Design review of the part built by this model. Coordinates are the model's own, in mm. A direction names the side the tool comes from. Give positions to 0.01 mm unless a question says otherwise; leave off trailing zeros. Loops run counter-clockwise (first coordinate to the right, second up) from the corner with the lowest first, then second, coordinate; pieces in that order, holes last. Notation, with made-up numbers: (-17.5, 32.25) -> (34.5, 32.25) arc R19 cw to (34.5, 62.25) -> close; hole circle Ø7 at (77.25, 4.25). An arc over 180 degrees is marked (long way). Answer in a Markdown table with one row per item. Add a question column.
(1) Draft analysis for pull direction X (two halves, no side actions). For faces 1 (the flat face through (9.15, 0, 1)), 2 (the flat face through (-0.394, -5.406, 0.74)), 3 (the flat face through (0, -12.3, 1)), state which applies: +X half, -X half, draft (parallel to the pull), parting line (faces both ways), or undercut.
(2) Consider section B-B on z = 0.4. Write out the cut boundary in (x, y).
(3) For line 1 (Y direction, x = 0.75, z = 1.35); line 2 (X direction, y = -6.5, z = 1.3), list the stretches that pass through material, from the lowest coordinate up.
(4) For faces 4 (the flat face through (1.494, -6.506, 0.74)), 5 (the flat face through (0, 0, 0)), list the 3-axis set-ups (+Z, -Z, +X, -X, +Y, -Y) from which the entire face can be reached by the end or side of a thin tool; tool diameter is ignored.
(5) Consider section A-A on x = -0.5. Write out the cut boundary in (y, z), then the cut area to 3 significant figures.
(6) Consider section C-C on y = -8. Write out the cut boundary in (x, z), then the cut area to 3 significant figures.
from build123d import *

# Parameters (mm, degrees)
EXTRUDE_3_DEPTH = 1.5


with BuildPart() as part:
    # Эскиз2 → Бобышка-Вытянуть3 (new body)
    with BuildSketch(Plane(origin=(0, 0, 0), x_dir=(-1, 0, 0), z_dir=(0, 0, 1))):
        Polygon((9.15, -11.885786438), (9.15, 11.885786438), (8.735786438, 12.3), (-8.735786438, 12.3), (-9.15, 11.885786438), (-9.15, -11.885786438), (-8.735786438, -12.3), (8.735786438, -12.3), align=None)
        Polygon((0, 8.5), (-0.8, 8.285640646), (-1.385640646, 7.7), (-1.6, 6.9), (-1.385640646, 6.1), (-0.8, 5.514359354), (0, 5.3), (0.8, 5.514359354), (1.385640646, 6.1), (1.6, 6.9), (1.385640646, 7.7), (0.8, 8.285640646), align=None, mode=Mode.SUBTRACT)
    extrude(amount=EXTRUDE_3_DEPTH)


solid = part.part
Values follow:
| question | item | result |
|---|---|---|
| 1 | face 1 | +X half |
| 1 | face 2 | undercut |
| 1 | face 3 | draft |
| 2 | outline | (-9.15, -11.89) -> (-8.74, -12.3) -> (8.74, -12.3) -> (9.15, -11.89) -> (9.15, 11.89) -> (8.74, 12.3) -> (-8.74, 12.3) -> (-9.15, 11.89) -> close; hole (-1.6, -6.9) -> (-1.39, -7.7) -> (-0.8, -8.29) -> (0, -8.5) -> (0.8, -8.29) -> (1.39, -7.7) -> (1.6, -6.9) -> (1.39, -6.1) -> (0.8, -5.51) -> (0, -5.3) -> (-0.8, -5.51) -> (-1.39, -6.1) -> close |
| 3 | line 1 | -12.3 to -8.3, -5.5 to 12.3 |
| 3 | line 2 | -9.15 to -1.49, 1.49 to 9.15 |
| 4 | face 4 | +Z, -Z |
| 4 | face 5 | -Z, +X, -X, +Y, -Y |
| 5 | outline | (-12.3, 0) -> (-8.37, 0) -> (-8.37, 1.5) -> (-12.3, 1.5) -> close; (-5.43, 0) -> (12.3, 0) -> (12.3, 1.5) -> (-5.43, 1.5) -> close |
| 5 | area | 32.5 mm2 |
| 6 | outline | (-9.15, 0) -> (-1.09, 0) -> (-1.09, 1.5) -> (-9.15, 1.5) -> close; (1.09, 0) -> (9.15, 0) -> (9.15, 1.5) -> (1.09, 1.5) -> close |
| 6 | area | 24.2 mm2 |
